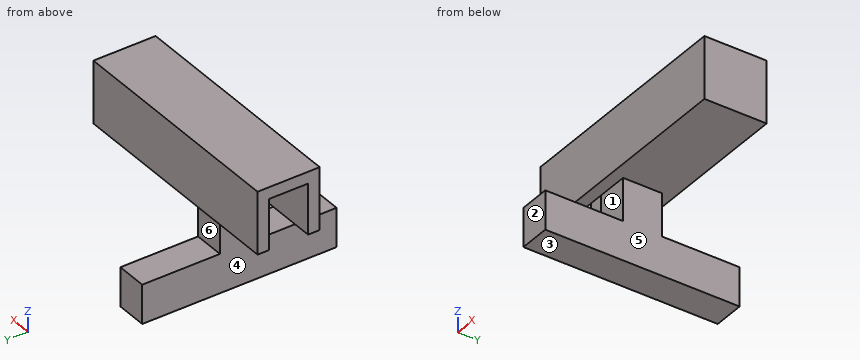
from build123d import *

# Parameters (mm, degrees)
SKETCH056_W     = 4
SKETCH056_H     = 4
PAD031_DEPTH    = 15
SKETCH057_W     = 2.5
SKETCH057_H     = 3.25
POCKET027_DEPTH = 4.5
PAD035_DEPTH    = 2


with BuildPart() as part:
    # Sketch056 → Pad031 (new body)
    with BuildSketch(Plane.YZ.offset(157)):
        with Locations((-60.5, 15.5)):
            Rectangle(SKETCH056_W, SKETCH056_H)
    extrude(amount=-PAD031_DEPTH)

    # Sketch057 (on Face6 of Pad031) → Pocket027 (cut)
    with BuildSketch(Plane(origin=(142, 0, 0), x_dir=(0, 1, 0), z_dir=(-1, 0, 0))):
        with Locations((-60.5, -15.125)):
            Rectangle(SKETCH057_W, SKETCH057_H)
    extrude(amount=-POCKET027_DEPTH, mode=Mode.SUBTRACT)

    # Sketch062 (on Face22 of Chamfer001) → Pad035 (join)
    with BuildSketch(Plane(origin=(146.5, 0, 0), x_dir=(0, -1, 0), z_dir=(-1, 0, 0))):
        Polygon((61.75, 13.5), (61.75, 10.75), (66.75, 10.75), (66.75, 8.25), (54.25, 8.25), (54.25, 10.75), (59.25, 10.75), (59.25, 13.5), align=None)
    extrude(amount=-PAD035_DEPTH)


solid = part.part
Can you work these out from the model? Positions are in its coordinate system, mm. Face numbers are marked on the shaded views. A direction names the side the tool comes from. Give positions to 0.01 mm unless a question says otherwise; leave off trailing zeros. Write each loop counter-clockwise with the first axis right and the second up, starting at its lowest first coordinate (ties: lowest second). Pieces come first, ordered by that corner, then holes. Notation, with made-up numbers: M 67.25,-23.75 L 80.25,-23.75 A16 ccw 80.25,-14.75 Z; hole C 61.25,23.25 d1. An arc over 180 degrees is marked long. Answer in a Markdown table with one row per item. Add a question column.
Item 1: For pin 1 Ø0.6 at (x, y) = (147.5, -63.5) entering from +Z; pin 2 Ø3 at (x, z) = (151.5, 15.5) entering from +Y; pin 3 Ø4 at (y, z) = (-58, 10.5) entering from +X, each with a flat end and sliding along its axis, tell me the tip position at first contact or that it passes through.
Item 2: Imagine slicing it at B-B, the plane y = -61.5. Write out the boundary of the cut face in (x, z), plus the area to 3 significant figures.
Item 3: Imagine slicing it at A-A, the plane x = 145. Write out the boundary of the cut face in (y, z).
Item 4: On a 3-axis mill with a long thin cutter (end or side, diameter ignored), from which of +Z, -Z, +X, -X, +Y, -Y can I reach the whole of each face in a straight line? I mean the marked faces 4, 5 and 6. Say none if no direction works.
Item 5: We'd pull the mould along Z, two halves only. Please class the marked faces 1, 2 and 3: released by +Z, released by -Z, zero draft, split by the parting line, or undercut.
Item 6: Imagine slicing it at D-D, the plane x = 147. Write out the boundary of the cut face in (y, z), plus the area to 3 significant figures.
Item 7: Please list where these lines run through material, in increasing order: L1, parallel to Z at x = 152, y = -61; L2, parallel to X at y = -59.5, z = 11; L3, parallel to Y at x = 148, z = 17.25.
Item 8: Imagine slicing it at C-C, the plane z = 10.5. Write out the boundary of the cut face in (x, y).
Evaluation:
| question | item | result |
|---|---|---|
| 1 | pin 1 | stops at z = 10.75 |
| 1 | pin 2 | stops at y = -58.5 |
| 1 | pin 3 | stops at x = 148.5 |
| 2 | outline | M 142,16.75 L 146.5,16.75 L 146.5,8.25 L 148.5,8.25 L 148.5,13.5 L 157,13.5 L 157,17.5 L 142,17.5 Z |
| 2 | area | 55.9 mm² |
| 3 | outline | M -62.5,13.5 L -61.75,13.5 L -61.75,16.75 L -59.25,16.75 L -59.25,13.5 L -58.5,13.5 L -58.5,17.5 L -62.5,17.5 Z |
| 4 | face 4 | -Z, -X |
| 4 | face 5 | -Z, +X, +Y, -Y |
| 4 | face 6 | +X, -X, +Y |
| 5 | face 1 | undercut |
| 5 | face 2 | zero draft |
| 5 | face 3 | released by -Z |
| 6 | outline | M -66.75,8.25 L -54.25,8.25 L -54.25,10.75 L -59.25,10.75 L -59.25,13.5 L -58.5,13.5 L -58.5,17.5 L -62.5,17.5 L -62.5,13.5 L -61.75,13.5 L -61.75,10.75 L -66.75,10.75 Z |
| 6 | area | 54.1 mm² |
| 7 | L1 | z = 13.5 to 17.5 |
| 7 | L2 | x = 146.5 to 148.5 |
| 7 | L3 | y = -62.5 to -58.5 |
| 8 | outline | M 146.5,-66.75 L 148.5,-66.75 L 148.5,-54.25 L 146.5,-54.25 Z |
